For this review, take the finished solid that the model builds, in its own axes (mm). A direction names the side the tool comes from. Round coordinates to 2 decimals unless told otherwise and drop trailing zeros. Loops run counter-clockwise (first coordinate to the right, second up) from the corner with the lowest first, then second, coordinate; pieces in that order, holes last. Notation, with made-up numbers: (67.25, 2.5) -> (114.25, 2.5) arc R20 ccw to (114.25, 27.5) -> close; hole circle Ø3 at (56.5, 67). An arc over 180 degrees is marked (long way). One line per question, with ' | ' between items. Start each with the question number.
1. For faces 4 (the face through (2.343, 17.847, 1.479)), 5 (the face through (-18, 3, 0)), list the 3-axis set-ups (+Z, -Z, +X, -X, +Y, -Y) from which the entire face can be reached by the end or side of a thin tool; tool diameter is ignored.
2. Draft analysis for pull direction X (two halves, no side actions). For faces 1 (the face through (-9, -15, 12)), 2 (the face through (9.139, 14.334, 13.479)), 3 (the face through (0, -12, 3)), state which applies: pulls with the +X half, pulls with the -X half, needs draft (parallel to the pull), parting line crosses it, or undercut.
3. Consider section A-A (x = 0). Write out the cut boundary in (y, z).
4. For pin 1 Ø5 at (y, z) = (-1.5, 2) entering from -X; pin 2 Ø5 at (x, z) = (-15, 8.5) entering from -Y; pin 3 Ø11 at (x, y) = (8, -4) entering from -Z; pin 4 Ø4 at (x, z) = (-6.5, 3.5) entering from -Y, all flat-tipped, find the tip position at first contact; note any pin that passes through.
5. Consider section D-D (x = 16). Write out the cut boundary in (y, z), and give its area (3 significant figures).
6. Wall thickness on line 1 along Y through (x, z) = (0, 9.5); line 2 along Y through (x, z) = (0, 1.15); line 3 along Z through (x, y) = (10, -12): over which ranges is each line inside the solid? List them lowest first.
7. Consider section C-C (z = 1). Write out the cut boundary in (x, y).
```python
from build123d import *

# Parameters (mm, degrees)
SKETCH_1_R          = 20
EXTRUDE_1_DEPTH     = 18
CUT_EXTRUDE_START   = -3
SKETCH_2_R          = 20
CUT_EXTRUDE_1_DEPTH = 3
SKETCH_5_R          = 20
SKETCH_5_R_2        = 17
CUT_EXTRUDE_4_DEPTH = 3
SKETCH_6_R          = 11.25
CUT_EXTRUDE_5_DEPTH = 50
SKETCH_7_R          = 18
CUT_EXTRUDE_6_DEPTH = 3


with BuildPart() as part:
    # 草图1 → 拉伸1 (new body)
    with BuildSketch(Plane.XY):
        Circle(SKETCH_1_R)
    extrude(amount=EXTRUDE_1_DEPTH)

    # 草图2 → 切除-拉伸1 (cut)
    with BuildSketch(Plane.XY.offset(18).offset(CUT_EXTRUDE_START)):
        Circle(SKETCH_2_R)
    extrude(amount=CUT_EXTRUDE_1_DEPTH, mode=Mode.SUBTRACT)

    # 草图5 → 切除-拉伸4 (cut)
    with BuildSketch(Plane.XY.offset(15).offset(CUT_EXTRUDE_START)):
        Circle(SKETCH_5_R)
        Circle(SKETCH_5_R_2, mode=Mode.SUBTRACT)
    extrude(amount=CUT_EXTRUDE_4_DEPTH, mode=Mode.SUBTRACT)

    # 草图6 → 切除-拉伸5 (cut)
    with BuildSketch(Plane(origin=(0, 0, 0), x_dir=(-1, 0, 0), z_dir=(0, 0, -1))):
        Circle(SKETCH_6_R)
    extrude(amount=-CUT_EXTRUDE_5_DEPTH, mode=Mode.SUBTRACT)

    # 草图7 → 切除-拉伸6 (cut)
    with BuildSketch(Plane(origin=(0, 0, 0), x_dir=(-1, 0, 0), z_dir=(0, 0, -1))):
        Circle(SKETCH_7_R)
    extrude(amount=-CUT_EXTRUDE_6_DEPTH, mode=Mode.SUBTRACT)


solid = part.part
```
Answer block:
1) face 4: -Z | face 5: -Z, +X, -X, +Y, -Y
2) face 1: needs draft | face 2: parting line crosses it | face 3: undercut
3) outline: (-20, 0) -> (-18, 0) -> (-18, 3) -> (-11.25, 3) -> (-11.25, 15) -> (-17, 15) -> (-17, 12) -> (-20, 12) -> close; (11.25, 3) -> (18, 3) -> (18, 0) -> (20, 0) -> (20, 12) -> (17, 12) -> (17, 15) -> (11.25, 15) -> close
4) pin 1: stops at x = -20 | pin 2: stops at y = -15.61 | pin 3: stops at z = 3 | pin 4: stops at y = -19.49
5) outline: (-12, 0) -> (-8.25, 0) -> (-8.25, 3) -> (8.25, 3) -> (8.25, 0) -> (12, 0) -> (12, 12) -> (5.74, 12) -> (5.74, 15) -> (-5.74, 15) -> (-5.74, 12) -> (-12, 12) -> close | area: 273 mm2
6) line 1: y = -20 to -11.25, 11.25 to 20 | line 2: y = -20 to -18, 18 to 20 | line 3: z = 3 to 15
7) outline: circle Ø40 at (0, 0); hole circle Ø36 at (0, 0)
